CAD build for the part. Positions are in the model's coordinates, mm. A direction names the side the tool comes from. Round coordinates to 2 decimals unless told otherwise and drop trailing zeros. Order: outer loops, then holes, each group sorted by start corner. A loop starts at its lowest first (then second) coordinate and runs counter-clockwise, first axis right, second up. Notation, with made-up numbers: (24, -39.5) -> (72, -39.5) arc R24 ccw to (72, -8.5) -> close; hole circle Ø11 at (77, -10.75). An arc over 180 degrees is marked (long way). Return JSON: item names as keys, results as strings. Group by question number.
Q1. Cut at D-D (z = 11.5). Write the cut outline in (x, y), then the cut area to 3 significant figures.
Q2. Cut at C-C (x = -4.25). Write the cut outline in (y, z).
Q3. Which spindle directions (+Z, -Z, +X, -X, +Y, -Y) get a long thin tool onto all of the face, cutting with end or side? Do faces 1 (the flat face through (4, 1, 12.018)), 2 (the flat face through (4, 1, 15.518)), 3 (the flat face through (4, 1, 5.018)), 4 (the flat face through (-4, 0, 2)). Say none if no direction does.
Q4. Mould opens along Z. For faces 5 (the flat face through (5.23, 1, 14)), 6 (the cylindrical face through (-4.42, 1.48, 15.08)), 7 (the flat face through (-2, 1, -14.982)) say: +Z half, -Z half, draft (parallel to the pull), parting line (faces both ways), or undercut.
Q5. Cut at A-A (x = 3). Write the cut outline in (y, z).
Q6. Probe line 1 along X through (y, z) = (1, -10); line 2 along Z through (x, y) = (3, 2.85); line 3 along Z through (x, y) = (-6, 1.6). List the from-to ranges inside material, lowest first.
Q7. Cut at B-B (y = 1.7). Write the cut outline in (x, z), then the cut area to 3 significant figures.
Q8. Flat gauge pins, fed straight in: pin 1 (1.5 mm diameter, centred on y = 2, z = 3.5, fed in from +X); pin 2 (3 mm diameter, centred on x = -4.77, z = -9.98, fed in from -Y); pin 3 (0.9 mm diameter, centred on x = 4, y = 1, fed in from -Z); pin 4 (0.9 mm diameter, centred on x = 3.5, y = 1, fed in from +Z). Where does each tip first touch, or does it go through?
Autodesk Inventor part; units mm, degrees
ref_plane "YZ Plane" through (0, 0, 0) normal (1, 0, 0) x (0, 1, 0)
ref_plane "XZ Plane" through (0, 0, 0) normal (0, 1, 0) x (-1, 0, 0)
ref_plane "XY Plane" through (0, 0, 0) normal (0, 0, 1) x (1, 0, 0)
sketch "Sketch1" plane through (0, 0, 0) normal (0, 1, 0) x (-1, 0, 0)
  circle A0 centre (4.7704, 13.5183) radius 1.6
  circle A1 centre (4.7704, -9.9817) radius 1.6
  line L0 (-5.2296, 5.0183) -> (-2.2296, 5.0183)
  line L1 (-5.2296, 15.5183) -> (-2.2296, 15.5183)
  line L2 (-5.2296, 8.5183) -> (-2.2296, 8.5183)
  line L3 (-5.2296, 12.0183) -> (-2.2296, 12.0183)
  line L4 (-5.2296, 5.0183) -> (-5.2296, 8.5183)
  line L5 (-5.2296, 12.0183) -> (-5.2296, 15.5183)
  line L6 (-2.2296, 15.5183) -> (-2.2296, 18.5183)
  line L7 (-2.2296, 5.0183) -> (-2.2296, -7.9817)
  line L8 (-2.2296, 8.5183) -> (-2.2296, 12.0183)
  line L9 (-2.2296, 18.5183) -> (4.7704, 18.5183)
  arc A2 (9.7704, 13.5183) -> (4.7704, 18.5183) centre (4.7704, 13.5183) ccw
  line L10 (9.7704, 13.5183) -> (9.7704, -4.9817)
  arc A3 (4.7704, -14.9817) -> (9.7704, -9.9817) centre (4.7704, -9.9817) ccw
  line L11 (4.7704, -14.9817) -> (-0.2296, -14.9817)
  arc A4 (-2.2296, -12.9817) -> (-0.2296, -14.9817) centre (-0.2296, -12.9817) ccw
  line L12 (4.7704, -4.9817) -> (4.7704, -9.9817)
  line L13 (-2.2296, -7.9817) -> (-2.2296, -12.9817)
  line L14 (9.7704, -4.9817) -> (9.7704, -9.9817)
  point P0 (0, 0)
  dimension "d2" = 5
extrude "Extrusion1" add sketch "Sketch1" along normal blind 3
properties part number "camMountBracket"
Solution:
{
 "1": {"outline": "(-9.77, 0) -> (2.23, 0) -> (2.23, 3) -> (-9.77, 3) -> close", "area": "36.0 mm²"},
 "2": {"outline": "(0, -14.98) -> (3, -14.98) -> (3, -11.49) -> (0, -11.49) -> close; (0, -8.47) -> (3, -8.47) -> (3, 12.01) -> (0, 12.01) -> close; (0, 15.03) -> (3, 15.03) -> (3, 18.52) -> (0, 18.52) -> close"},
 "3": {"face 1": "+X, +Y, -Y", "face 2": "+Z, +X, +Y, -Y", "face 3": "-Z, +X, +Y, -Y", "face 4": "+Z, -Z, +X, -X, -Y"},
 "4": {"face 5": "draft", "face 6": "undercut", "face 7": "-Z half"},
 "5": {"outline": "(0, 5.02) -> (3, 5.02) -> (3, 8.52) -> (0, 8.52) -> close; (0, 12.02) -> (3, 12.02) -> (3, 15.52) -> (0, 15.52) -> close"},
 "6": {"line 1": "x = -9.77 to -6.37, -3.17 to 2.23", "line 2": "z = 5.02 to 8.52, 12.02 to 15.52", "line 3": "z = -14.83 to -11.01, -8.96 to 12.49, 14.54 to 18.36"},
 "7": {"outline": "(-9.77, -9.98) arc R5 ccw to (-4.77, -14.98) -> (0.23, -14.98) arc R2 ccw to (2.23, -12.98) -> (2.23, 5.02) -> (5.23, 5.02) -> (5.23, 8.52) -> (2.23, 8.52) -> (2.23, 12.02) -> (5.23, 12.02) -> (5.23, 15.52) -> (2.23, 15.52) -> (2.23, 18.52) -> (-4.77, 18.52) arc R5 ccw to (-9.77, 13.52) -> close; hole circle Ø3.2 at (-4.77, -9.98); hole circle Ø3.2 at (-4.77, 13.52)", "area": "395 mm²"},
 "8": {"pin 1": "stops at x = 2.23", "pin 2": "passes through", "pin 3": "stops at z = 5.02", "pin 4": "stops at z = 15.52"}
}
